CAD build for the part. Positions are in the model's coordinates, mm. A direction names the side the tool comes from. Give positions to 0.01 mm unless a question says otherwise; leave off trailing zeros. Order: outer loops, then holes, each group sorted by start corner. A loop starts at its lowest first (then second) coordinate and runs counter-clockwise, first axis right, second up.
Item 1: Band-saw the part on C-C on y = 10.5. Give the cut face in (x, z).
Item 2: Two-plate mould, pull along Z, no slides. Class faces 4 (the cylindrical face through (-16.059, 12.758, -3.566)), 5 (the flat face through (-7, 0, -7)), 6 (the cylindrical face through (-5.3, 24, -6.9)), 7 (the cylindrical face through (0.856, -3.978, -2.164)): released by +Z, released by -Z, zero draft, split by the parting line, or undercut.
Item 3: Flat gauge pins, fed straight in: P1, Ø4, axis at x = 8.5, z = 10, coming from the -Y side; P2, Ø1.5, axis at y = 26, z = 6.5, coming from the +X side; P3, Ø12, axis at y = 0.5, z = -7, coming from the -X side. Where does each tip first touch, or does it go through?
Item 4: Band-saw the part on A-A on y = 24. Give the cut face in (x, z), plus the area to 3 significant figures.
Item 5: Which spindle directions (+Z, -Z, +X, -X, +Y, -Y) get a long thin tool onto all of the face, cutting with end or side? Do faces 1 (the flat face through (0, 34.3, 0)), 2 (the cylindrical face through (0.401, -13.831, -1.273)), 3 (the flat face through (-4, 23.2, 0)). Say none if no direction does.
Item 6: Wall check: L1, parallel to X at y = 24.3, z = 0; L2, parallel to X at y = 2.05, z = 0; L3, parallel to Y at x = 1, z = 10.5. Give the ranges that are in metal, low to high.
```python
from build123d import *

# Parameters (mm, degrees)
SKETCH1_R           = 16.45
BOSS_EXTRUDE1_DEPTH = 25.85
SKETCH2_R           = 8.7
CUT_EXTRUDE1_DEPTH  = 2.65
SKETCH3_R           = 3.15
BOSS_EXTRUDE2_DEPTH = 11.1
CUT_EXTRUDE2_START  = -3.2
SKETCH4_R           = 8.7
CUT_EXTRUDE2_DEPTH  = 3.2
SKETCH5_R           = 1.335
BOSS_EXTRUDE3_DEPTH = 19.12
SKETCH6_R           = 2.825
BOSS_EXTRUDE4_DEPTH = 14.56
FILLET1_R           = 1
CUT_EXTRUDE9_START  = -14.56
CUT_EXTRUDE9_DEPTH  = 14.56
CIRPATTERN3_COUNT   = 8
SKETCH16_R          = 1.835
BOSS_EXTRUDE6_DEPTH = 15


with BuildPart() as part:
    # Sketch1 → Boss-Extrude1 (new body)
    with BuildSketch(Plane(origin=(0, 0, 0), x_dir=(1, 0, 0), z_dir=(0, 1, 0))):
        with Locations(Location((0, 0, 0), (0, 0, 270))):
            Circle(SKETCH1_R)
    extrude(amount=BOSS_EXTRUDE1_DEPTH)

    # Sketch2 → Cut-Extrude1 (cut)
    with BuildSketch(Plane(origin=(0, 25.85, 0), x_dir=(1, 0, 0), z_dir=(0, 1, 0))):
        with Locations(Location((0, 0, 0), (0, 0, 270))):
            Circle(SKETCH2_R)
    extrude(amount=-CUT_EXTRUDE1_DEPTH, mode=Mode.SUBTRACT)

    # Sketch3 → Boss-Extrude2 (add)
    with BuildSketch(Plane(origin=(0, 23.2, 0), x_dir=(1, 0, 0), z_dir=(0, 1, 0))):
        with Locations(Location((0, 0, 0), (0, 0, 270))):
            Circle(SKETCH3_R)
    extrude(amount=BOSS_EXTRUDE2_DEPTH)

    # Sketch4 → Cut-Extrude2 (cut)
    with BuildSketch(Plane.XZ.offset(CUT_EXTRUDE2_START)):
        with Locations(Location((0, 0, 0), (0, 0, 90))):
            Circle(SKETCH4_R)
    extrude(amount=CUT_EXTRUDE2_DEPTH, mode=Mode.SUBTRACT)

    # Sketch5 → Boss-Extrude3 (add)
    with BuildSketch(Plane.XZ.offset(-3.2)):
        with Locations(Location((0, 0, 0), (0, 0, 270))):
            Circle(SKETCH5_R)
    extrude(amount=BOSS_EXTRUDE3_DEPTH)

    # Sketch6 → Boss-Extrude4 (add)
    with BuildSketch(Plane.XZ.offset(-3.2)):
        with Locations(Location((0, 0, 0), (0, 0, 270))):
            Circle(SKETCH6_R)
    extrude(amount=BOSS_EXTRUDE4_DEPTH)

    # Fillet1
    fillet1_edges = [part.edges().sort_by_distance(p)[0] for p in [
        (0, 0, -8.7),
        (0, 0, -16.45),
        (0, 25.85, -16.45),
        (0, 25.85, -8.7),
    ]]
    fillet(fillet1_edges, radius=FILLET1_R)

    # Sketch15 → Cut-Extrude9 (cut)
    with BuildSketch(Plane.XZ.offset(11.36).offset(CUT_EXTRUDE9_START)):
        with BuildLine():
            ThreePointArc((1.372148642, 2.469379093), (0.431099526, 2.791913), (-0.563406151, 2.768248275))
            ThreePointArc((-0.563406151, 2.768248275), (-0.104815557, 2.083529636), (0.203723139, 1.319364196))
            ThreePointArc((0.203723139, 1.319364196), (0.728385952, 1.954874919), (1.372148642, 2.469379093))
        make_face()
    cut_extrude9 = extrude(amount=CUT_EXTRUDE9_DEPTH, mode=Mode.SUBTRACT)

    # CirPattern3: Cut-Extrude9 ×8 about axis
    cirpattern3_axis = Axis((0, 0, 0), (0, 1, 0))
    for i in range(1, CIRPATTERN3_COUNT):
        add(cut_extrude9.rotate(cirpattern3_axis, i * 360 / CIRPATTERN3_COUNT), mode=Mode.SUBTRACT)

    # Sketch16 → Boss-Extrude6 (add)
    with BuildSketch(Plane.XZ.offset(-3.2)):
        with Locations(Location((0, 0, 0), (0, 0, 89.500330008))):
            Circle(SKETCH16_R)
    extrude(amount=BOSS_EXTRUDE6_DEPTH)


solid = part.part
```
The answers:
1. outline: circle Ø32.9 at (0, 0)
2. face 4: split by the parting line
2. face 5: zero draft
2. face 6: undercut
2. face 7: undercut
3. P1: stops at y = 0
3. P2: stops at x = 15.12
3. P3: stops at x = -16.42
4. outline: circle Ø32.9 at (0, 0); circle Ø6.3 at (0, 0); hole circle Ø17.4 at (0, 0)
4. area: 644 mm2
5. face 1: +Z, -Z, +X, -X, +Y
5. face 2: -Y
5. face 3: +Y
6. L1: x = -16.45 to -8.7, -3.15 to 3.15, 8.7 to 16.45
6. L2: x = -16.45 to -8.7, -1.87 to 1.87, 8.7 to 16.45
6. L3: y = 0 to 25.85
